Study the drawing (mm; zero at the part's minimum x, y, z) and answer. Coordinates: 2 decimals unless noted, no trailing zeros. Order: outer loops, then holes, each group sorted by start corner. A loop starts at its lowest first (then second) coordinate and runs counter-clockwise, first axis right, second up. Notation, with made-up numbers: M 12,-1 L 21,-1 A21 cw 21,16 Z; hole C 67.25,18.5 d2. An arc over 180 degrees is marked long. Use a Markdown table: item, result. Add a question column.
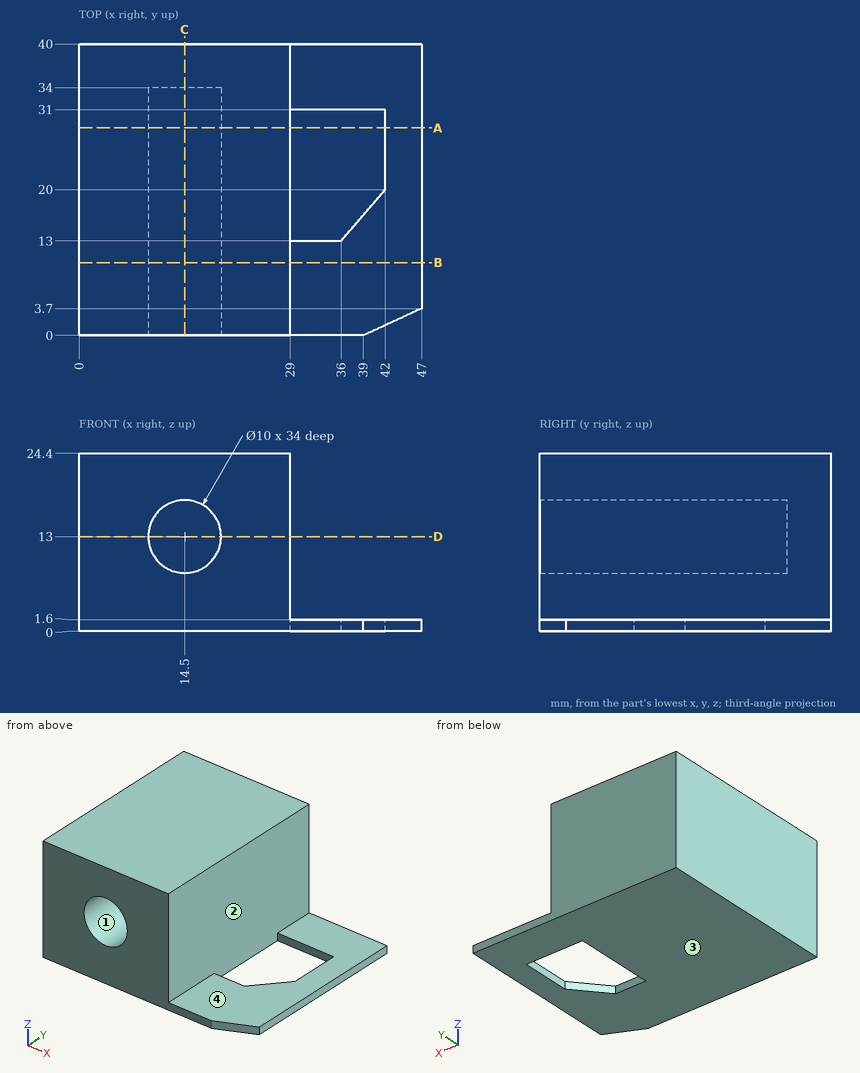
(1) A cutting plane is placed at D-D on z = 13. Write down the section's boundary in (x, y), plus the area to 3 significant figures.
(2) The mould has two halves that part along Z. Classify the marked faces 1, 2, 3 and 4: pulls with the +Z half, pulls with the -Z half, needs draft (parallel to the pull), parting line crosses it, or undercut.
(3) Given P1, Ø7.5, axis at y = 27.5, z = 14.5, coming from the +X side; P2, Ø6, axis at x = 14.5, z = 13, coming from the -Y side; P3, Ø20, axis at x = 41, y = 25.5, coming from the +Z side; P4, Ø1.5, axis at x = 31.5, y = 24, coming from the -Z side, each flat-ended and moving along its own axis, determine where each tip first touches the part or whether it passes through.
(4) A cutting plane is placed at B-B on y = 10. Write down the section's boundary in (x, z).
(5) A cutting plane is placed at A-A on y = 28.5. Write down the section's boundary in (x, z), plus the area to 3 significant figures.
(6) Straight lines are drawn through the part: line 1 (X direction, y = 7.5, z = 13); line 2 (Y direction, x = 33.5, z = 1.5); line 3 (X direction, y = 37, z = 16.5). For each, find the intervals that lie inside material, in ascending order.
(7) A cutting plane is placed at C-C on x = 14.5. Write down the section's boundary in (y, z), plus the area to 3 significant figures.
From the geometry:
| question | item | result |
|---|---|---|
| 1 | outline | M 0,0 L 9.5,0 L 9.5,34 L 19.5,34 L 19.5,0 L 29,0 L 29,40 L 0,40 Z |
| 1 | area | 820 mm2 |
| 2 | face 1 | undercut |
| 2 | face 2 | needs draft |
| 2 | face 3 | pulls with the -Z half |
| 2 | face 4 | pulls with the +Z half |
| 3 | P1 | stops at x = 29 |
| 3 | P2 | stops at y = 34 |
| 3 | P3 | stops at z = 1.6 |
| 3 | P4 | passes through |
| 4 | outline | M 0,0 L 47,0 L 47,1.6 L 29,1.6 L 29,24.4 L 0,24.4 Z; hole C 14.5,13 d10 |
| 5 | outline | M 0,0 L 29,0 L 29,24.4 L 0,24.4 Z; M 42,0 L 47,0 L 47,1.6 L 42,1.6 Z; hole C 14.5,13 d10 |
| 5 | area | 637 mm2 |
| 6 | line 1 | x = 0 to 9.5, 19.5 to 29 |
| 6 | line 2 | y = 0 to 13, 31 to 40 |
| 6 | line 3 | x = 0 to 29 |
| 7 | outline | M 0,0 L 40,0 L 40,24.4 L 0,24.4 L 0,18 L 34,18 L 34,8 L 0,8 Z |
| 7 | area | 636 mm2 |
